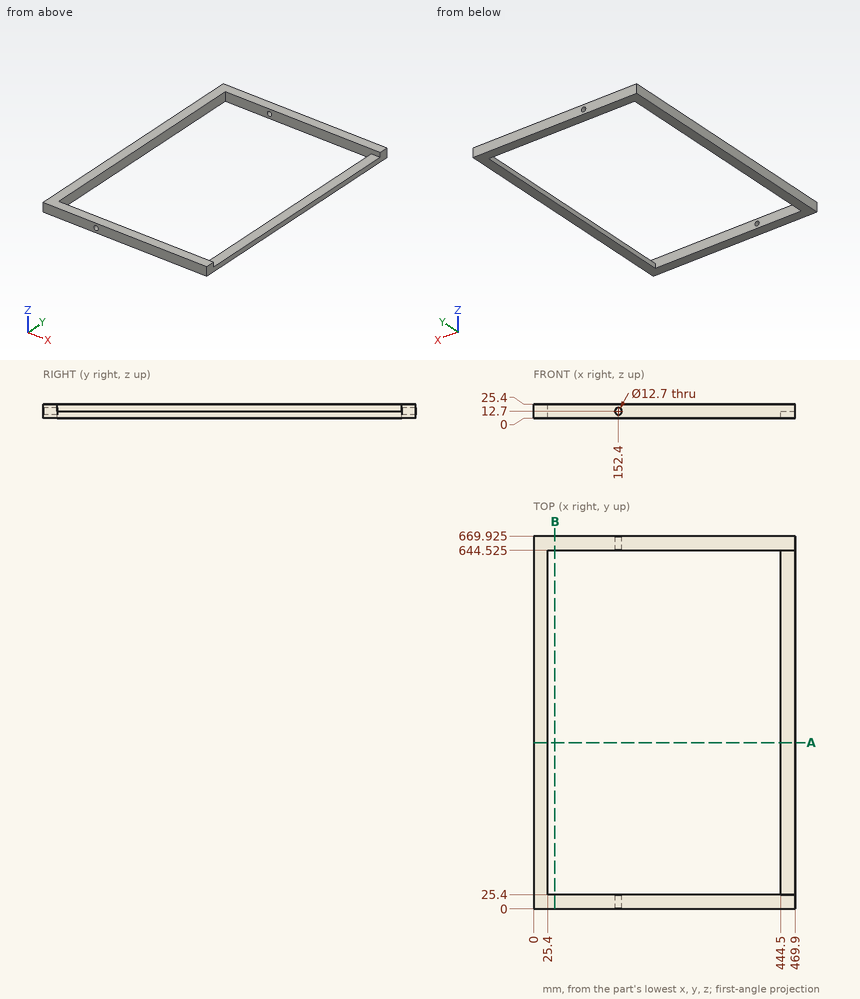
Drawing for the job (mm, zero at the part's lowest x, y, z). Give positions to 0.01 mm unless a question says otherwise; leave off trailing zeros. Loops run counter-clockwise (first coordinate to the right, second up) from the corner with the lowest first, then second, coordinate; pieces in that order, holes last.
1) Probe line 1 along Y through (x, z) = (352, 16.5) (3 decimals); line 2 along Z through (x, y) = (152.4, 660.25); line 3 along X through (y, z) = (424, 9). List the from-to ranges inside material, lowest first.
Values follow:
line 1: y = 0 to 25.4, 644.525 to 669.925
line 2: z = 0 to 6.35, 19.05 to 25.4
line 3: x = 0 to 25.4, 444.5 to 469.9
2) Band-saw the part on B-B on x = 38. List the corners of the cut face in (y, z) (3 decimals).
Values follow:
outline: (0, 0) - (25.4, 0) - (25.4, 25.4) - (0, 25.4) - close; (644.525, 0) - (669.925, 0) - (669.925, 25.4) - (644.525, 25.4) - close
3) Band-saw the part on A-A on y = 298.5. List the corners of the cut face in (x, z), then the cut area to 3 significant figures.
Values follow:
outline: (0, 0) - (25.4, 0) - (25.4, 25.4) - (0, 25.4) - close; (444.5, 0) - (469.9, 0) - (469.9, 12.7) - (444.5, 12.7) - close
area: 968 mm2
4) Drop flat-ended pins along their axis: P1, Ø4, axis at y = 277.5, z = 7.5, coming from the -X side; P2, Ø20.5, axis at x = 456, y = 263, coming from the +Z side. Give the stop position or say it passes through.
Values follow:
P1: stops at x = 0
P2: stops at z = 12.7
